```python
from build123d import *

# Parameters (mm, degrees)
F1_DEPTH  = 22.352
F2_DEPTH  = 3.175
F4_DEPTH  = 1143
F6_R      = 6.35
F6_R_2    = 3.175
F7_DEPTH  = 3.175
F8_R      = 6.35
F8_R_2    = 3.175
F9_DEPTH  = 3.175
F10_DEPTH = 28.5637839421
F11_R     = 10.922
F12_R     = 22.35199


# Not quite as in the source:
# - a fillet or chamfer is up to 0.001 mm smaller than in the source, because OpenCascade refuses the exact size


with BuildPart() as f1:
    # F0 (on Front) → F1 (new body, symmetric)
    with BuildSketch(Plane.XZ):
        Polygon((-14.5947370299, 9.652), (-33.6447370299, 42.6475678842), (-42.0036142272, 37.8215678842), (-20.1673218281, 0), (69.9872629701, 0), (69.9872629701, 9.652), (10.8052629701, 9.652), align=None)
    extrude(amount=F1_DEPTH, both=True)

    # F0 (on Front) → F2 (join, symmetric)
    with BuildSketch(Plane.XZ):
        Polygon((10.8052629701, 9.652), (-33.6447370299, 42.6475678842), (-14.5947370299, 9.652), align=None)
    extrude(amount=F2_DEPTH, both=True)

    # F3 (on face) → F4 (cut)
    with BuildSketch(Plane.XY.offset(9.652)):
        with BuildLine():
            ThreePointArc((23.5052629701, 9.652), (16.6802683181, 6.824994652), (13.8532629701, 0))
            Line((13.8532629701, 0), (23.5052629701, 0))
            Line((23.5052629701, 0), (26.5532629701, 0))
            ThreePointArc((26.5532629701, 0), (27.1079902762, 4.9488187589), (28.7446379798, 9.652))
            Line((28.7446379798, 9.652), (23.5052629701, 9.652))
        make_face()
        with BuildLine():
            Line((23.5052629701, 0), (13.8532629701, 0))
            ThreePointArc((13.8532629701, 0), (16.6802683181, -6.824994652), (23.5052629701, -9.652))
            Line((23.5052629701, -9.652), (28.7446379798, -9.652))
            ThreePointArc((28.7446379798, -9.652), (27.1079902762, -4.9488187589), (26.5532629701, 0))
            Line((26.5532629701, 0), (23.5052629701, 0))
        make_face()
        with BuildLine():
            ThreePointArc((28.7446379798, 9.652), (27.1079902762, 4.9488187589), (26.5532629701, 0))
            ThreePointArc((26.5532629701, 0), (27.1079902762, -4.9488187589), (28.7446379798, -9.652))
            Line((28.7446379798, -9.652), (48.9052629701, -9.652))
            ThreePointArc((48.9052629701, -9.652), (58.5572629701, 0), (48.9052629701, 9.652))
            Line((48.9052629701, 9.652), (28.7446379798, 9.652))
        make_face()
    extrude(amount=-F4_DEPTH, mode=Mode.SUBTRACT)

    # F6 (on face) → F7 (cut)
    with BuildSketch(Plane(origin=(-6.7666141738, 0, -3.9067065147), x_dir=(0, 1, 0), z_dir=(0.8660254038, 0, 0.5))):
        with Locations((11.43, 42.8342457123)):
            Circle(F6_R)
        with Locations((11.43, 42.8342457123)):
            Circle(F6_R_2, mode=Mode.SUBTRACT)
    extrude(amount=-F7_DEPTH, mode=Mode.SUBTRACT)

    # F8 (on face) → F9 (cut)
    with BuildSketch(Plane(origin=(-6.7666141738, 0, -3.9067065147), x_dir=(0, 1, 0), z_dir=(0.8660254038, 0, 0.5))):
        with Locations((-11.43, 42.8342457123)):
            Circle(F8_R)
        with Locations((-11.43, 42.8342457123)):
            Circle(F8_R_2, mode=Mode.SUBTRACT)
    extrude(amount=-F9_DEPTH, mode=Mode.SUBTRACT)

    # F10 (cut, through all): faces of the model
    f10_faces = [f1.faces().sort_by_distance(p)[0] for p in [
        (-28.1837370299, -11.43, 33.1888384241),
        (-28.1837370299, 11.43, 33.1888384241),
    ]]
    extrude(f10_faces, amount=-F10_DEPTH, mode=Mode.SUBTRACT)

    # F11
    f11_edges = [f1.edges().sort_by_distance(p)[0] for p in [
        (-37.824176, -22.352, 40.234568),
        (-37.824176, 22.352, 40.234568),
    ]]
    fillet(f11_edges, radius=F11_R)

    # F12 (radius 22.352 in the source; OpenCascade refuses exactly that, so slightly less here)
    f12_edges = [f1.edges().sort_by_distance(p)[0] for p in [
        (69.987263, 22.352, 4.826),
        (69.987263, -22.352, 4.826),
    ]]
    fillet(f12_edges, radius=F12_R)


solid = f1.part
```
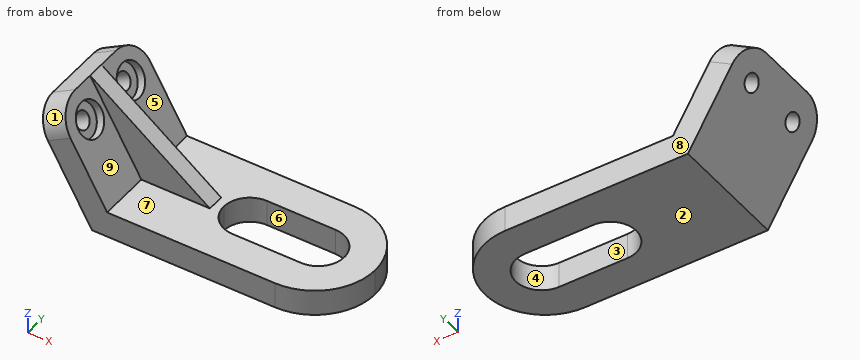
The model under review builds one solid part; all positions refer to its coordinate system, in mm. Face numbers are marked on the shaded views. A direction names the side the tool comes from. Give positions to 0.01 mm unless a question says otherwise; leave off trailing zeros. Order: outer loops, then holes, each group sorted by start corner. A loop starts at its lowest first (then second) coordinate and runs counter-clockwise, first axis right, second up. Notation, with made-up numbers: (-14, 43) - (33, 43) arc R22 cw to (33, 62) - close; hole circle Ø7 at (-3, 31.25). An arc over 180 degrees is marked (long way). Use CSV: the item, a comma, the result in double quotes. Start each with the question number.
Q1. To check wall thickness, follow line 1 along Y through (x, z) = (37.5, 2); line 2 along Z through (x, y) = (33.5, 16); line 3 along Y through (x, z) = (-13, 17) (3 decimals). State the ranges of each line that lie inside material, in increasing order. Write a range as [from, to].
Q2. We need section A-A, the plane x = 52. Write out the cut boundary in (y, z).
Q3. The part is to be moulded in two halves that separate along Y. For the marked faces 1, 2, 3 and 4, say which applies: +Y half, -Y half, draft (parallel to the pull), parting line (faces both ways), or undercut.
Q4. We need section C-C, the plane z = 11.5. Write out the cut boundary in (x, y) (3 decimals), and give its area (3 significant figures).
Q5. We need section B-B, the plane y = 2. Write out the cut boundary in (x, z).
Q6. We need section D-D, the plane x = -8.5. Write out the cut boundary in (y, z) (3 decimals).
Q7. Clearance check with flat-ended pins moving along their axes: pin 1 Ø10 at (x, y) = (17, -8.5) entering from +Z; pin 2 Ø16.5 at (x, z) = (-6, 26) entering from +Y (3 decimals); pin 3 Ø8 at (y, z) = (1, 8) entering from -X. State where each tip first meets the part, or that it passes through.
Q8. Tool access review of the marked faces 5, 6, 7, 8 and 9: name each direction out of +Z, -Z, +X, -X, +Y, -Y from which nothing blocks a thin tool from reaching the whole face with its end or side.
Outcome:
1,line 1,"y = [-22.35, -9.65], [9.65, 22.35]"
1,line 2,"z = [0, 9.65]"
1,line 3,"y = [-3.175, 3.175]"
2,outline,"(-21.92, 0) - (-9.14, 0) - (-9.14, 9.65) - (-21.92, 9.65) - close; (9.14, 0) - (21.92, 0) - (21.92, 9.65) - (9.14, 9.65) - close"
3,face 1,"-Y half"
3,face 2,"draft"
3,face 3,"undercut"
3,face 4,"undercut"
4,outline,"(-26.807, -22.352) - (-15.662, -22.352) - (-15.662, -3.175) - (8.316, -3.175) - (8.316, 3.175) - (-15.662, 3.175) - (-15.662, 22.352) - (-26.807, 22.352) - close"
4,area,"650 mm^2"
5,outline,"(-42, 37.82) - (-20.17, 0) - (14.06, 0) - (14.06, 9.65) - (10.81, 9.65) - (-33.64, 42.65) - close; (58.35, 0) - (69.9, 0) - (69.9, 9.65) - (58.35, 9.65) - close"
6,outline,"(-22.352, 0) - (22.352, 0) - (22.352, 9.652) - (3.175, 9.652) - (3.175, 23.982) - (-3.175, 23.982) - (-3.175, 9.652) - (-22.352, 9.652) - close"
7,pin 1,"stops at z = 9.65"
7,pin 2,"stops at y = 3.175"
7,pin 3,"stops at x = -27.1"
8,face 5,"+Z, +X, +Y"
8,face 6,"+Z, -Z"
8,face 7,"+Z, +X"
8,face 8,"+Z, -Z, +X, -X, +Y"
8,face 9,"+Z, +X, -Y"
